from build123d import *

# Parameters (mm, degrees)
F0_R      = 98
F1_DEPTH  = 1284.5
F2_R      = 98
F2_R_2    = 50
F3_DEPTH  = 200
F4_SIZE   = 40
F5_R      = 5
F8_DEPTH  = 30
F9_R      = 6.75
F9_R_2    = 7.5
F10_DEPTH = 10.001


# Not quite as in the source:
# - a pattern or mirror of a feature is missing from the dataset's text; its kind, count and spacing are read off the source's solid


with BuildPart() as f1:
    # F0 (on Top) → F1 (new body, symmetric)
    with BuildSketch(Plane.XY):
        Circle(F0_R)
    extrude(amount=F1_DEPTH, both=True)

    # F2 (on face) → F3 (cut)
    with BuildSketch(Plane(origin=(0, 0, -1284.5), x_dir=(1, 0, 0), z_dir=(0, 0, -1))):
        Circle(F2_R)
        Circle(F2_R_2, mode=Mode.SUBTRACT)
    extrude(amount=-F3_DEPTH, mode=Mode.SUBTRACT)

    # F4
    f4_edges = [f1.edges().sort_by_distance(p)[0] for p in [
        (-50, 0, -1084.5),
    ]]
    chamfer(f4_edges, length=F4_SIZE)

    # F5
    f5_edges = [f1.edges().sort_by_distance(p)[0] for p in [
        (-50, 0, -1284.5),
        (-98, 0, 1284.5),
    ]]
    fillet(f5_edges, radius=F5_R)

    # F7 (on offset) → F8 (join)
    with BuildSketch(Plane(origin=(0, 0, -1064.5), x_dir=(1, 0, 0), z_dir=(0, 0, -1))):
        Polygon((76.2233031652, -72.2150126676), (65.2159465136, -73.14971169), (132.6794919243, -190), (-132.6794919243, -190), (-65.2159465136, -73.14971169), (-76.2233031652, -72.2150126676), (-144.2264973081, -190), (-200, -190), (-200, -200), (-150, -200), (150, -200), (200, -200), (200, -190), (144.2264973081, -190), align=None)
        with BuildLine():
            ThreePointArc((-65.2159465136, -73.14971169), (0, 98), (65.2159465136, -73.14971169))
            Line((65.2159465136, -73.14971169), (76.2233031652, -72.2150126676))
            ThreePointArc((76.2233031652, -72.2150126676), (0, 105), (-76.2233031652, -72.2150126676))
            Line((-76.2233031652, -72.2150126676), (-65.2159465136, -73.14971169))
        make_face()
    f8 = extrude(amount=-F8_DEPTH)

    # F8_copies: F8 across plane
    add(f8.mirror(Plane.XY.offset(-314.5)))

    # F9 (on face) → F10 (cut, through all)
    with BuildSketch(Plane.XZ.offset(-190)):
        with Locations((-172.1132486541, -1049.5)):
            Circle(F9_R)
        with Locations((176.858574152, -1049.5)):
            Circle(F9_R_2)
    f10 = extrude(amount=-F10_DEPTH, mode=Mode.SUBTRACT)

    # F10_copies: F10 across plane
    add(f10.mirror(Plane.XY.offset(-314.5)), mode=Mode.SUBTRACT)


solid = f1.part
Can you work these out from the model? Positions are in its coordinate system, mm. A direction names the side the tool comes from. Give positions to 0.01 mm unless a question says otherwise; leave off trailing zeros. Loops run counter-clockwise (first coordinate to the right, second up) from the corner with the lowest first, then second, coordinate; pieces in that order, holes last. Notation, with made-up numbers: M -26,-11 L 29,-11 A30 cw 29,16 Z; hole C -32.5,18 d1. An arc over 180 degrees is marked long. One line per item, written item: value.
1) I'm going to push flat-ended pins straight in: pin 1 (9 mm diameter, centred on x = -183, z = 416, fed in from -Y); pin 2 (8 mm diameter, centred on y = 23.5, z = 757.5, fed in from -X); pin 3 (4 mm diameter, centred on x = 16, y = 60.5, fed in from -Z). Where does each tip first touch, or does it pass through?
Geometry check:
pin 1: stops at y = 190
pin 2: stops at x = -96.04
pin 3: stops at z = -1113.92
2) On a 3-axis mill with a long thin cutter (end or side, diameter ignored), from which of +Z, -Z, +X, -X, +Y, -Y can I reach the whole of each face in a straight line? I mean faces 4 (the face through (110.7, 131.93, -1049.71)), 5 (the face through (98.5, 130.8, -1049.7)), 6 (the face through (73, 81, 405.5)), 7 (the face through (73, 81, 435.5)). Say none if no direction works.
Geometry check:
face 4: +Z, -Z, +X
face 5: +Z, -Z
face 6: none
face 7: +Z
3) Imagine slicing it at C-C on z = -917. Write out the boundary of the cut face in (x, y).
Geometry check:
outline: C 0,0 d196
4) Imagine slicing it at A-A on x = 0. Count the separate pieces of the cut face and the enclosed holes in it, and give its area (3 significant figures).
Geometry check:
separate pieces: 3
enclosed holes: 0
area: 487,000 mm²
5) Thinking about a two-plate mould opening in Y: for faces 1 (the face through (-1, 1, -1284.5)), 2 (the face through (110.7, 131.93, 420.71)), 3 (the face through (47.69, -15.02, -1203.08)), which applies, +Y half, -Y half, draft (parallel to the pull), parting line (faces both ways), or undercut?
Geometry check:
face 1: draft
face 2: undercut
face 3: parting line
6) Please list where these lines run through material, in increasing order: line 1 (X direction, y = 197, z = -1049); line 2 (X direction, y = 194.5, z = 420.5); line 3 (Z direction, x = -139, y = 182.5).
Geometry check:
line 1: x = -200 to -178.84, -165.38 to 169.38, 184.34 to 200
line 2: x = -200 to -178.86, -165.36 to 169.36, 184.36 to 200
line 3: z = -1064.5 to -1034.5, 405.5 to 435.5
7) Imagine slicing it at B-B on y = 146.5. Write out the boundary of the cut face in (x, z).
Geometry check:
outline: M -119.11,-1064.5 L -107.56,-1064.5 L -107.56,-1034.5 L -119.11,-1034.5 Z; M -119.11,405.5 L -107.56,405.5 L -107.56,435.5 L -119.11,435.5 Z; M 107.56,-1064.5 L 119.11,-1064.5 L 119.11,-1034.5 L 107.56,-1034.5 Z; M 107.56,405.5 L 119.11,405.5 L 119.11,435.5 L 107.56,435.5 Z
